```python
from build123d import *

# Parameters (mm, degrees)
F1_DEPTH      = 37.5
F3_R          = 3.125
F4_DEPTH      = 37.5
F4_DEPTH_BACK = 37.5
F5_W          = 12.7266719937
F5_H          = 25
F6_DEPTH      = 71.001
F6_DEPTH_BACK = 5.126
F2_R          = 3
F7_DEPTH      = 71.001


with BuildPart() as f1:
    # F0 (on Front) → F1 (new body, symmetric)
    with BuildSketch(Plane.XZ):
        with BuildLine():
            ThreePointArc((64.3155620097, -9.4078947368), (0, -65), (-64.3155620097, -9.4078947368))
            ThreePointArc((-64.3155620097, -9.4078947368), (-68.0064440401, -2.6779462302), (-75.1997340421, 0))
            Line((-75.1997340421, 0), (-110, 0))
            Line((-110, 0), (-110, -6))
            Line((-110, -6), (-75.1997340421, -6))
            ThreePointArc((-75.1997340421, -6), (-71.9300567685, -7.2172482865), (-70.2523831183, -10.2763157895))
            ThreePointArc((-70.2523831183, -10.2763157895), (0, -71), (70.2523831183, -10.2763157895))
            ThreePointArc((70.2523831183, -10.2763157895), (71.9300567685, -7.2172482865), (75.1997340421, -6))
            Line((75.1997340421, -6), (110, -6))
            Line((110, -6), (110, 0))
            Line((110, 0), (75.1997340421, 0))
            ThreePointArc((75.1997340421, 0), (68.0064440401, -2.6779462302), (64.3155620097, -9.4078947368))
        make_face()
    extrude(amount=F1_DEPTH, both=True)

    # F3 (on Front) → F4 (join, two sides)
    with BuildSketch(Plane.XZ) as f4_sk:
        with BuildLine():
            ThreePointArc((110, -3.971), (110.4913325801, -3.253734436), (111.3376547749, -3.4527729648))
            ThreePointArc((111.3376547749, -3.4527729648), (119.9038999403, 1.851415772), (110, 0))
            Line((110, 0), (110, -3.971))
        make_face()
        with Locations((115.125, 0)):
            Circle(F3_R, mode=Mode.SUBTRACT)
    extrude(amount=F4_DEPTH)
    extrude(f4_sk.sketch, amount=-F4_DEPTH_BACK)

    # F5 (on Top) → F6 (cut, two sides)
    with BuildSketch(Plane.XY) as f6_sk:
        with Locations((116.3633359969, 0)):
            Rectangle(F5_W, F5_H)
    extrude(amount=-F6_DEPTH, mode=Mode.SUBTRACT)
    extrude(f6_sk.sketch, amount=F6_DEPTH_BACK, mode=Mode.SUBTRACT)

    # F2 (on face) → F7 (cut, through all)
    with BuildSketch(Plane.XY):
        with Locations((-90, 17.5)):
            Circle(F2_R)
        with Locations((-90, -17.5)):
            Circle(F2_R)
    extrude(amount=-F7_DEPTH, mode=Mode.SUBTRACT)


solid = f1.part
```
The model under review builds one solid part; all positions refer to its coordinate system, in mm. A direction names the side the tool comes from. Give positions to 0.01 mm unless a question says otherwise; leave off trailing zeros. Order: outer loops, then holes, each group sorted by start corner. A loop starts at its lowest first (then second) coordinate and runs counter-clockwise, first axis right, second up. Notation, with made-up numbers: (37, 44) - (53, 44) arc R20 ccw to (53, 52) - close; hole circle Ø7 at (49, 15.25). An arc over 180 degrees is marked (long way). Use CSV: the item, a comma, the result in double quotes. Start each with the question number.
Q1. The part is to be moulded in two halves that separate along X. For faces 6 (the flat face through (110, -1, -4)), 7 (the cylindrical face through (71.89, -0.52, -7.25)), 8 (the flat face through (115.1, -12.5, -3.3)), 9 (the cylindrical face through (-93, -17.4, -3)), say which applies: +X half, -X half, draft (parallel to the pull), parting line (faces both ways), or undercut.
Q2. We need section B-B, the plane z = -44.5. Write out the cut boundary in (x, y), and give its area (3 significant figures).
Q3. We need section C-C, the plane y = -17.5. Write out the cut boundary in (x, z) (3 decimals), and give its area (3 significant figures).
Q4. We need section D-D, the plane z = -62.5. Write out the cut boundary in (x, y).
Q5. Tool access review of faces 1 (the flat face through (-93, -1, -6)), 2 (the cylindrical face through (119.972, 24.825, 1.665)), 3 (the flat face through (93, -1, 0)), 4 (the cylindrical face through (-67.924, -0.525, -2.75)), 5 (the flat face through (92, -1, -6)): name each direction out of +Z, -Z, +X, -X, +Y, -Y from which nothing blocks a thin tool from reaching the whole face with its end or side.
Q6. Clearance check with flat-ended pins moving along their axes: pin 1 Ø12 at (x, y) = (-61.5, 25) entering from -Z; pin 2 Ø17.5 at (x, y) = (100, 17) entering from +Z; pin 3 Ø8 at (x, y) = (-90, -17.5) entering from -Z. State where each tip first meets the part, or that it passes through.
Q7. We need section A-A, the plane x = -90. Write out the cut boundary in (y, z).
Q8. To check wall thickness, follow line 1 along Y through (x, z) = (-90, -2.75); line 2 along X through (y, z) = (17, -1); line 3 along X through (y, z) = (-17, -4). State the ranges of each line that lie inside material, in increasing order. Write a range as [from, to].
Outcome:
1,face 6,"undercut"
1,face 7,"+X half"
1,face 8,"draft"
1,face 9,"undercut"
2,outline,"(-55.32, -37.5) - (-47.38, -37.5) - (-47.38, 37.5) - (-55.32, 37.5) - close; (47.38, -37.5) - (55.32, -37.5) - (55.32, 37.5) - (47.38, 37.5) - close"
2,area,"1,190 mm^2"
3,outline,"(-110, -6) - (-93, -6) - (-93, 0) - (-110, 0) - close; (-87, -6) - (-75.2, -6) arc R5 cw to (-70.252, -10.276) arc R71 ccw to (70.252, -10.276) arc R5 cw to (75.2, -6) - (110, -6) - (110, -3.971) arc R0.769 cw to (111.338, -3.453) arc R5.125 ccw (long way) to (110, 0) - (75.2, 0) arc R11 ccw to (64.316, -9.408) arc R65 cw to (-64.316, -9.408) arc R11 ccw to (-75.2, 0) - (-87, 0) - close; hole circle Ø6.25 at (115.125, 0)"
3,area,"1,730 mm^2"
4,outline,"(-33.69, -37.5) - (-17.85, -37.5) - (-17.85, 37.5) - (-33.69, 37.5) - close; (17.85, -37.5) - (33.69, -37.5) - (33.69, 37.5) - (17.85, 37.5) - close"
5,face 1,"-Z, -X, +Y, -Y"
5,face 2,"+Y, -Y"
5,face 3,"+Z, -X, +Y, -Y"
5,face 4,"+Z, +Y, -Y"
5,face 5,"-Z, +X, +Y, -Y"
6,pin 1,"stops at z = -44.28"
6,pin 2,"stops at z = 0"
6,pin 3,"stops at z = -6"
7,outline,"(-37.5, -6) - (-20.5, -6) - (-20.5, 0) - (-37.5, 0) - close; (-14.5, -6) - (14.5, -6) - (14.5, 0) - (-14.5, 0) - close; (20.5, -6) - (37.5, -6) - (37.5, 0) - (20.5, 0) - close"
8,line 1,"y = [-37.5, -20.5], [-14.5, 14.5], [20.5, 37.5]"
8,line 2,"x = [-110, -92.96], [-87.04, -70.62], [70.62, 112.16], [118.09, 120.15]"
8,line 3,"x = [-110, -92.96], [-87.04, -66.71], [66.71, 110], [111.92, 118.33]"
